```python
from build123d import *

# Parameters (mm, degrees)
SKETCH_2_W          = 2.2
SKETCH_2_H          = 4.2
CUT_EXTRUDE_1_DEPTH = 4.2


with BuildPart() as part:
    # 草图1 → 旋转2 (revolve)
    with BuildSketch(Plane(origin=(0, 0, 0), x_dir=(1, 0, 0), z_dir=(0, 1, 0))):
        with BuildLine():
            Line((-5, -6.244997998), (0, -6.244997998))
            Line((0, -6.244997998), (0, 8))
            ThreePointArc((0, 8), (-7.548509256, 2.649529771), (-5, -6.244997998))
        make_face()
    revolve(axis=Axis((0, 0, 6.244997998), (0, 0, -1)))

    # 草图2 → 切除-拉伸1 (cut)
    with BuildSketch(Plane.XY.offset(6.244997998)):
        Rectangle(SKETCH_2_W, SKETCH_2_H)
    extrude(amount=-CUT_EXTRUDE_1_DEPTH, mode=Mode.SUBTRACT)


solid = part.part
```
Model file for the job. Use its own axes, mm. Round coordinates to 2 decimals unless told otherwise and drop trailing zeros. Write each loop counter-clockwise with the first axis right and the second up, starting at its lowest first coordinate (ties: lowest second). Pieces come first, ordered by that corner, then holes. Notation, with made-up numbers: M 45.25,-18.5 L 98.25,-18.5 A25 cw 98.25,1.5 Z; hole C 9.25,-29 d7. An arc over 180 degrees is marked long. Put each result on its own line as item: value.
Item 1: Mould opens along Y. For faces 1 (the flat face through (1.1, 0, 4)), 2 (the flat face through (-2, 0, 6.245)) say: +Y half, -Y half, draft (parallel to the pull), parting line (faces both ways), or undercut.
Responses:
face 1: undercut
face 2: draft
Item 2: Cut at B-B (x = -3). List the corners of the cut face in (y, z) (3 decimals).
Responses:
outline: M -4,6.245 A7.416 ccw long 4,6.245 Z
Item 3: Cut at D-D (z = 4.25). List the corners of the cut face in (x, y), and give its area (3 significant figures).
Responses:
outline: C 0,0 d13.56; hole M -1.1,-2.1 L 1.1,-2.1 L 1.1,2.1 L -1.1,2.1 Z
area: 135 mm²
Item 4: Probe L1, parallel to X at y = 1.5, z = 2.75; L2, parallel to Z at x = 0, y = -0.25 (3 decimals); L3, parallel to Y at x = 3.5, z = -3.5. List the from-to ranges inside material, lowest first. Write a range as from..to.
Responses:
L1: -7.36..-1.1, 1.1..7.36
L2: -7.996..2.045
L3: -6.28..6.28
Item 5: Cut at A-A (z = 2.5). List the corners of the cut face in (x, y), and give its area (3 significant figures).
Responses:
outline: C 0,0 d15.2; hole M -1.1,-2.1 L 1.1,-2.1 L 1.1,2.1 L -1.1,2.1 Z
area: 172 mm²
Item 6: Flat gauge pins, fed straight in: P1, Ø1, axis at x = 5.5, z = 3.5, coming from the -Y side; P2, Ø1, axis at y = 0, z = -5.5, coming from the +X side (3 decimals); P3, Ø8, axis at y = -4, z = -4.5, coming from the -X side. Where does each tip first touch, or does it go through?
Responses:
P1: y = -5.27
P2: x = 6.245
P3: x = -7.74
Item 7: Cut at C-C (y = -1.25). List the corners of the cut face in (x, z) (3 decimals).
Responses:
outline: M -4.841,6.245 A7.902 ccw long 4.841,6.245 L 1.1,6.245 L 1.1,2.045 L -1.1,2.045 L -1.1,6.245 Z
